from build123d import *

# Parameters (mm, degrees)
SKETCH1_W                  = 250
SKETCH1_H                  = 344
SKETCH1_R                  = 23.5
SKETCH1_R_2                = 8.5
SKETCH1_R_3                = 12.5
BOSS_EXTRUDE1_DEPTH        = 12
M5_TAPPED_HOLE1_AT_2_COUNT = 2
M5_TAPPED_HOLE1_AT_2_PITCH = 46
M6_TAPPED_HOLE1_D          = 5
M5_TAPPED_HOLE2_D          = 4.2
M5_TAPPED_HOLE2_DEPTH      = 15
M5_TAPPED_HOLE2_TIP        = 1.2618073
M5_TAPPED_HOLE3_AT_2_COUNT = 2
M5_TAPPED_HOLE3_AT_2_PITCH = 55
M5_TAPPED_HOLE3_AT_3_COUNT = 2
M5_TAPPED_HOLE3_AT_3_PITCH = 110


with BuildPart() as part:
    # Sketch1 → Boss-Extrude1 (new body)
    with BuildSketch(Plane.XY):
        with Locations((0, 122)):
            Rectangle(SKETCH1_W, SKETCH1_H)
        with Locations((-80, 244)):
            Circle(SKETCH1_R, mode=Mode.SUBTRACT)
        with Locations((80, 244)):
            Circle(SKETCH1_R, mode=Mode.SUBTRACT)
        with Locations((-100, 83)):
            Circle(SKETCH1_R_2, mode=Mode.SUBTRACT)
        with Locations((100, 83)):
            Circle(SKETCH1_R_2, mode=Mode.SUBTRACT)
        with Locations((-30, 0)):
            Circle(SKETCH1_R_3, mode=Mode.SUBTRACT)
        with Locations((85, 0)):
            Circle(SKETCH1_R_3, mode=Mode.SUBTRACT)
    extrude(amount=BOSS_EXTRUDE1_DEPTH)

    # Sketch5 → M5 Tapped Hole1 (revolve, cut)
    with BuildSketch(Plane(origin=(-125, 282, 6), x_dir=(0, 0, 1), z_dir=(0, 1, 0))):
        Polygon((0, 0), (0, 16.2618073), (2.1, 15), (2.1, 0), align=None)
    m5_tapped_hole1 = revolve(axis=Axis((-131.35, 282, 6), (1, 0, 0)), mode=Mode.SUBTRACT)

    # M5 Tapped Hole1 at 2: M5 Tapped Hole1 ×2
    with Locations(*[(0, -i * M5_TAPPED_HOLE1_AT_2_PITCH, 0) for i in range(1, M5_TAPPED_HOLE1_AT_2_COUNT)]):
        add(m5_tapped_hole1, mode=Mode.SUBTRACT)

    # Mirror1: M5 Tapped Hole1 across plane
    add(m5_tapped_hole1.mirror(Plane(origin=(0, 0, 0), x_dir=(0, 0, 1), z_dir=(1, 0, 0))), mode=Mode.SUBTRACT)

    # Mirror1 copy 1 sketch → Mirror1 copy 1 (revolve, cut)
    with BuildSketch(Plane(origin=(125, 236, 6), x_dir=(0, 0, 1), z_dir=(0, 1, 0))):
        Polygon((0, 0), (0, -16.2618073), (2.1, -15), (2.1, 0), align=None)
    revolve(axis=Axis((131.35, 236, 6), (1, 0, 0)), mode=Mode.SUBTRACT)

    # M6 Tapped Hole1 (through all)
    with Locations(Plane.XY.offset(12)):
        with Locations((-105, 269), (-55, 269), (-55, 219), (-105, 219), (55, 219), (105, 219), (105, 269), (55, 269), (-55, 25), (-5, 25), (-5, -25), (-55, -25), (60, 25), (110, 25), (110, -25), (60, -25)):
            Hole(M6_TAPPED_HOLE1_D / 2)

    # M5 Tapped Hole2
    with Locations(Plane(origin=(0, -50, 0), x_dir=(-1, 0, 0), z_dir=(0, -1, 0))):
        with Locations((-113, -6), (-67, -6), (67, -6), (113, -6)):
            Hole(M5_TAPPED_HOLE2_D / 2, depth=M5_TAPPED_HOLE2_DEPTH)
            with Locations((0, 0, -(M5_TAPPED_HOLE2_DEPTH + M5_TAPPED_HOLE2_TIP / 2))):  # 118° drill point
                Cone(0, M5_TAPPED_HOLE2_D / 2, M5_TAPPED_HOLE2_TIP, mode=Mode.SUBTRACT)

    # Sketch19 → M5 Tapped Hole3 (revolve, cut)
    with BuildSketch(Plane(origin=(125, 97, 6), x_dir=(0, 0, -1), z_dir=(0, 1, 0))):
        Polygon((0, 0), (0, 16.2618073), (2.1, 15), (2.1, 0), align=None)
    m5_tapped_hole3 = revolve(axis=Axis((131.35, 97, 6), (-1, 0, 0)), mode=Mode.SUBTRACT)

    # M5 Tapped Hole3 at 2: M5 Tapped Hole3 ×2
    with Locations(*[(0, i * M5_TAPPED_HOLE3_AT_2_PITCH, 0) for i in range(1, M5_TAPPED_HOLE3_AT_2_COUNT)]):
        add(m5_tapped_hole3, mode=Mode.SUBTRACT)

    # M5 Tapped Hole3 at 3: M5 Tapped Hole3 ×2
    with Locations(*[(0, i * M5_TAPPED_HOLE3_AT_3_PITCH, 0) for i in range(1, M5_TAPPED_HOLE3_AT_3_COUNT)]):
        add(m5_tapped_hole3, mode=Mode.SUBTRACT)

    # Mirror2: M5 Tapped Hole3 across plane
    add(m5_tapped_hole3.mirror(Plane(origin=(0, 0, 0), x_dir=(0, 0, 1), z_dir=(1, 0, 0))), mode=Mode.SUBTRACT)

    # Mirror2 copy 1 sketch → Mirror2 copy 1 (revolve, cut)
    with BuildSketch(Plane(origin=(-125, 152, 6), x_dir=(0, 0, -1), z_dir=(0, 1, 0))):
        Polygon((0, 0), (0, -16.2618073), (2.1, -15), (2.1, 0), align=None)
    revolve(axis=Axis((-131.35, 152, 6), (-1, 0, 0)), mode=Mode.SUBTRACT)

    # Mirror2 copy 2 sketch → Mirror2 copy 2 (revolve, cut)
    with BuildSketch(Plane(origin=(-125, 207, 6), x_dir=(0, 0, -1), z_dir=(0, 1, 0))):
        Polygon((0, 0), (0, -16.2618073), (2.1, -15), (2.1, 0), align=None)
    revolve(axis=Axis((-131.35, 207, 6), (-1, 0, 0)), mode=Mode.SUBTRACT)


solid = part.part
Work out the finished part from the listing and answer in its coordinate system (mm). Round coordinates to 2 decimals unless told otherwise and drop trailing zeros. Write each loop counter-clockwise with the first axis right and the second up, starting at its lowest first coordinate (ties: lowest second). Pieces come first, ordered by that corner, then holes.
1) Given pin 1 Ø4 at (y, z) = (282, 6) entering from +X; pin 2 Ø3.5 at (x, z) = (113, 6) entering from -Y; pin 3 Ø3 at (x, y) = (-5, -25) entering from +Z, each flat-ended and moving along its own axis, determine where each tip first touches the part or whether it passes through.
2) A cutting plane is placed at A-A (y = 244). Give the vertices of the cut face in (x, z), plus the area to 3 significant figures.
3) A cutting plane is placed at C-C (y = 83). Give the vertices of the cut face in (x, z), plus the area to 3 significant figures.
4) The mould has two halves that part along Y. Classify faces 1 (the flat face through (125, 120, 6)), 2 (the cylindrical face through (91.51, 83.37, 5.92)), 3 (the flat face through (-2, -50, 6)): pulls with the +Y half, pulls with the -Y half, needs draft (parallel to the pull), parting line crosses it, or undercut.
5) A cutting plane is placed at B-B (x = -30). Give the vertices of the cut face in (y, z), plus the area to 3 significant figures.
6) A cutting plane is placed at D-D (x = -87). Give the vertices of the cut face in (y, z), plus the area to 3 significant figures.
7) Straight lines are drawn through the part: line 1 (Y direction, x = 117, z = 6); line 2 (X direction, y = 251, z = 8); line 3 (Y direction, x = 115, z = 6). For each, find the intervals that lie inside material, in ascending order.
Completed:
1. pin 1: stops at x = 109.94
1. pin 2: stops at y = -34.79
1. pin 3: passes through
2. outline: (-125, 0) - (-103.5, 0) - (-103.5, 12) - (-125, 12) - close; (-56.5, 0) - (56.5, 0) - (56.5, 12) - (-56.5, 12) - close; (103.5, 0) - (125, 0) - (125, 12) - (103.5, 12) - close
2. area: 1,870 mm2
3. outline: (-125, 0) - (-108.5, 0) - (-108.5, 12) - (-125, 12) - close; (-91.5, 0) - (91.5, 0) - (91.5, 12) - (-91.5, 12) - close; (108.5, 0) - (125, 0) - (125, 12) - (108.5, 12) - close
3. area: 2,590 mm2
4. face 1: needs draft
4. face 2: undercut
4. face 3: pulls with the -Y half
5. outline: (-50, 0) - (-12.5, 0) - (-12.5, 12) - (-50, 12) - close; (12.5, 0) - (294, 0) - (294, 12) - (12.5, 12) - close
5. area: 3,830 mm2
6. outline: (-50, 0) - (221.57, 0) - (221.57, 12) - (-50, 12) - close; (266.43, 0) - (294, 0) - (294, 12) - (266.43, 12) - close
6. area: 3,590 mm2
7. line 1: y = -50 to 94.9, 99.1 to 149.9, 154.1 to 204.9, 209.1 to 233.9, 238.1 to 279.9, 284.1 to 294
7. line 2: x = -125 to -102.43, -57.57 to 57.57, 102.43 to 125
7. line 3: y = -34.94 to 94.9, 99.1 to 149.9, 154.1 to 204.9, 209.1 to 233.9, 238.1 to 279.9, 284.1 to 294
